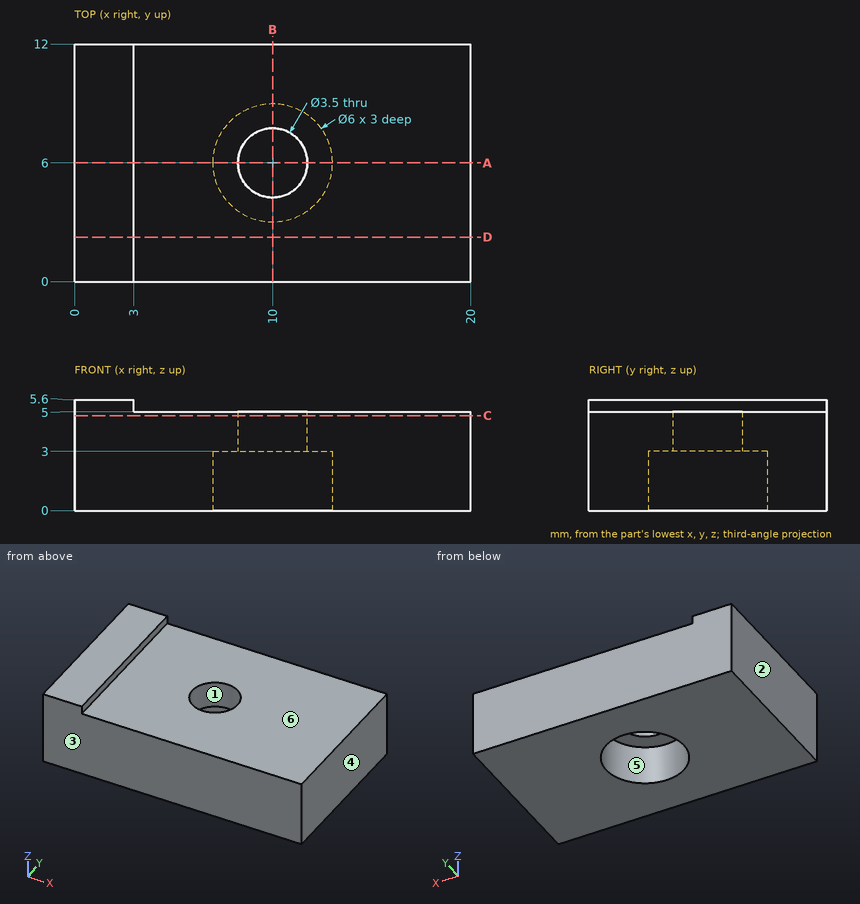
The drawing under review shows one solid part. Ordinate dimensions are in mm from its lowest x, y, z. A direction names the side the tool comes from. Give positions to 0.01 mm unless a question says otherwise; leave off trailing zeros. Write each loop counter-clockwise with the first axis right and the second up, starting at its lowest first coordinate (ties: lowest second). Pieces come first, ordered by that corner, then holes. Notation, with made-up numbers: (-2.75, -21) -> (26.25, -21) arc R29 cw to (26.25, 4) -> close; hole circle Ø7 at (33.25, 12). An arc over 180 degrees is marked (long way). Put each result on its own line as item: value.
(1) To check wall thickness, follow probe 1 along X at (y, z) = (6, 3.8); probe 2 along Y at (x, z) = (10, 4.05); probe 3 along Y at (x, z) = (10, 1.1). State the ranges of each line that lie inside material, in increasing order. Write a range as from..to.
Results are:
probe 1: 0..8.25, 11.75..20
probe 2: 0..4.25, 7.75..12
probe 3: 0..3, 9..12
(2) We need section D-D, the plane y = 2.25. Give the boundary of the cut face in (x, z).
Results are:
outline: (0, 0) -> (20, 0) -> (20, 5) -> (3, 5) -> (3, 5.6) -> (0, 5.6) -> close
(3) We need section B-B, the plane x = 10. Give the boundary of the cut face in (y, z).
Results are:
outline: (0, 0) -> (3, 0) -> (3, 3) -> (4.25, 3) -> (4.25, 5) -> (0, 5) -> close; (7.75, 3) -> (9, 3) -> (9, 0) -> (12, 0) -> (12, 5) -> (7.75, 5) -> close
(4) We need section C-C, the plane z = 4.8. Give the boundary of the cut face in (x, y), and give its area (3 significant figures).
Results are:
outline: (0, 0) -> (20, 0) -> (20, 12) -> (0, 12) -> close; hole circle Ø3.5 at (10, 6)
area: 230 mm²
(5) Tool access review of the marked faces 4, 5 and 6: name each direction out of +Z, -Z, +X, -X, +Y, -Y from which nothing blocks a thin tool from reaching the whole face with its end or side.
Results are:
face 4: +Z, -Z, +X, +Y, -Y
face 5: -Z
face 6: +Z, +X, +Y, -Y
(6) We need section A-A, the plane y = 6. Give the boundary of the cut face in (x, z).
Results are:
outline: (0, 0) -> (7, 0) -> (7, 3) -> (8.25, 3) -> (8.25, 5) -> (3, 5) -> (3, 5.6) -> (0, 5.6) -> close; (11.75, 3) -> (13, 3) -> (13, 0) -> (20, 0) -> (20, 5) -> (11.75, 5) -> close
(7) For pin 1 Ø0.7 at (y, z) = (8.5, 5.5) entering from +X; pin 2 Ø3 at (x, y) = (10, 5.5) entering from -Z; pin 3 Ø4 at (x, y) = (16, 9) entering from -Z, all flat-tipped, find the tip position at first contact; note any pin that passes through.
Results are:
pin 1: x = 3
pin 2: z = 3
pin 3: z = 0
(8) The part is to be moulded in two halves that separate along Y. For the marked faces 1, 2 and 3, say which applies: pulls with the +Y half, pulls with the -Y half, needs draft (parallel to the pull), parting line crosses it, or undercut.
Results are:
face 1: undercut
face 2: needs draft
face 3: pulls with the -Y half
